Read the model definition and answer for the solid it produces. Units are mm, in the model's axes. A direction names the side the tool comes from. Coordinates: 2 decimals unless noted, no trailing zeros. Order: outer loops, then holes, each group sorted by start corner. A loop starts at its lowest first (then second) coordinate and runs counter-clockwise, first axis right, second up. Notation, with made-up numbers: M -10,5.5 L 22,5.5 A18 cw 22,34.5 Z; hole C 9.5,64.5 d6. An arc over 180 degrees is marked long. Put each result on its own line as item: value.
from build123d import *

# Parameters (mm, degrees)
BOSS_EXTRUDE1_DEPTH     = 15
M2_5_CLEARANCE_HOLE1_D  = 2.9
CUT_EXTRUDE1_DEPTH      = 28.093587802
CUT_EXTRUDE1_DEPTH_BACK = 28.093587802
SKETCH3_R               = 4.365625
M2_CLEARANCE_HOLE1_D    = 2.4
SKETCH10_R              = 11.5
CUT_EXTRUDE3_DEPTH      = 1
FILLET1_R               = 1
FILLET2_R               = 3


with BuildPart() as part:
    # Sketch2 → Boss-Extrude1 (new, symmetric)
    with BuildSketch(Plane.XY):
        Polygon((0, 21.75), (0, -21.75), (10, -21.75), (10, -17.25), (4, -17.25), (4, 17.25), (10, 17.25), (10, 21.75), align=None)
    extrude(amount=BOSS_EXTRUDE1_DEPTH, both=True)

    # M2.5 Clearance Hole1 (through all)
    with Locations(Plane(origin=(0, -21.75, 0), x_dir=(-1, 0, 0), z_dir=(0, -1, 0))):
        with Locations((-7.2, -11), (-7.2, 11)):
            Hole(M2_5_CLEARANCE_HOLE1_D / 2)

    # Sketch3 → Cut-Extrude1 (cut, two sides: drawn at the far end of the back side and taken through both)
    with BuildSketch(Plane(origin=(4, 0, 0), x_dir=(0, 0, -1), z_dir=(1, 0, 0)).offset(-CUT_EXTRUDE1_DEPTH_BACK)):
        with Locations(Location((0, 0, 0), (0, 0, 90))):
            Circle(SKETCH3_R)
    extrude(amount=CUT_EXTRUDE1_DEPTH + CUT_EXTRUDE1_DEPTH_BACK, mode=Mode.SUBTRACT)

    # M2 Clearance Hole1 (through all)
    with Locations(Plane.ZY):
        with Locations((5.656854249, 5.656854249), (5.656854249, -5.656854249), (-5.656854249, -5.656854249), (-5.656854249, 5.656854249), (0, 0)):
            Hole(M2_CLEARANCE_HOLE1_D / 2)

    # Sketch10 → Cut-Extrude3 (cut)
    with BuildSketch(Plane.ZY):
        with Locations(Location((0, 0, 0), (0, 0, 270))):
            Circle(SKETCH10_R)
    extrude(amount=-CUT_EXTRUDE3_DEPTH, mode=Mode.SUBTRACT)

    # Fillet1
    fillet1_edges = [part.edges().sort_by_distance(p)[0] for p in [
        (4, 17.25, 0),
        (4, -17.25, 0),
    ]]
    fillet(fillet1_edges, radius=FILLET1_R)

    # Fillet2
    fillet2_edges = [part.edges().sort_by_distance(p)[0] for p in [
        (0, -21.75, 0),
        (0, 21.75, 0),
    ]]
    fillet(fillet2_edges, radius=FILLET2_R)


solid = part.part
Q1. Find section A-A on x = 9.25. Write down the section's boundary in (y, z), plus the area to 3 significant figures.
Answers below:
outline: M -21.75,-15 L -17.25,-15 L -17.25,15 L -21.75,15 Z; M 17.25,-15 L 21.75,-15 L 21.75,15 L 17.25,15 Z
area: 270 mm^2
Q2. For a pull along Y with two mould halves and no side action, classify faces 3 (the face through (8.539, 19.531, 11.555)), 4 (the face through (0.49, -6.18, 9.7)), 5 (the face through (0.9, -20.89, 0.21)) as +Y half, -Y half, draft (parallel to the pull), parting line (faces both ways), or undercut.
Answers below:
face 3: draft
face 4: undercut
face 5: -Y half
Q3. Find section B-B on y = 0. Write down the section's boundary in (x, z).
Answers below:
outline: M 0,-15 L 4,-15 L 4,-4.37 L 1,-4.37 L 1,-11.5 L 0,-11.5 Z; M 0,11.5 L 1,11.5 L 1,4.37 L 4,4.37 L 4,15 L 0,15 Z
Q4. Consider line 1 along Z through (x, y) = (7.2, -19.35); line 2 along Z through (x, y) = (0.4, 0); line 3 along Y through (x, z) = (6.5, 0). Determine where each line is inside the solid, lowest interval first.
Answers below:
line 1: z = -15 to -12.45, -9.55 to 9.55, 12.45 to 15
line 2: z = -15 to -11.5, 11.5 to 15
line 3: y = -21.75 to -17.25, 17.25 to 21.75
Q5. Find section C-C on x = 7.2. Write down the section's boundary in (y, z), plus the area to 3 significant figures.
Answers below:
outline: M -21.75,-15 L -17.25,-15 L -17.25,-12.45 L -21.75,-12.45 Z; M -21.75,-9.55 L -17.25,-9.55 L -17.25,9.55 L -21.75,9.55 Z; M -21.75,12.45 L -17.25,12.45 L -17.25,15 L -21.75,15 Z; M 17.25,-15 L 21.75,-15 L 21.75,-12.45 L 17.25,-12.45 Z; M 17.25,-9.55 L 21.75,-9.55 L 21.75,9.55 L 17.25,9.55 Z; M 17.25,12.45 L 21.75,12.45 L 21.75,15 L 17.25,15 Z
area: 218 mm^2
Q6. Given pin 1 (9 mm diameter, centred on y = 5.5, z = 4.5, fed in from +X), flat-ended and moving along its own axis, determine where the tip first touches the part or whether it passes through.
Answers below:
pin 1: stops at x = 4
Q7. A tool of negligible diameter and unlimited length cuts with its end or side. For faces 1 (the face through (7, 17.25, 0)), 2 (the face through (8.539, -19.469, 11.555)), from which of +Z, -Z, +X, -X, +Y, -Y can it reach the whole face along a straight path? Write none if from no direction.
Answers below:
face 1: +Z, -Z, +X
face 2: +Y, -Y
Q8. Find section D-D on z = 0. Write down the section's boundary in (x, y), plus the area to 3 significant figures.
Answers below:
outline: M 0,-18.75 A3 ccw 3,-21.75 L 10,-21.75 L 10,-17.25 L 5,-17.25 A1 cw 4,-16.25 L 4,-4.37 L 1,-4.37 L 1,-11.5 L 0,-11.5 Z; M 0,11.5 L 1,11.5 L 1,4.37 L 4,4.37 L 4,16.25 A1 cw 5,17.25 L 10,17.25 L 10,21.75 L 3,21.75 A3 ccw 0,18.75 Z
area: 175 mm^2
